Work out the finished part from the listing and answer in its coordinate system (mm). Give positions to 0.01 mm unless a question says otherwise; leave off trailing zeros. Loops run counter-clockwise (first coordinate to the right, second up) from the corner with the lowest first, then second, coordinate; pieces in that order, holes last. Notation, with made-up numbers: M 39,50 L 88,50 A6 cw 88,61 Z; hole C 6.5,1.25 d8. An arc over 180 degrees is marked long. Answer in a Markdown table with one row per item. Add a question column.
from build123d import *

# Parameters (mm, degrees)
F0_R     = 2.5
F0_R_2   = 1.5
F0_R_3   = 11
F1_DEPTH = 5


with BuildPart() as f1:
    # F0 (on Front) → F1 (new body)
    with BuildSketch(Plane.XZ):
        Polygon((-75, -140), (75, -140), (75, 140), (0, 140), (-75, -11.7), align=None)
        with Locations((-40, -120)):
            Circle(F0_R, mode=Mode.SUBTRACT)
        with Locations((-40, -38)):
            Circle(F0_R, mode=Mode.SUBTRACT)
        with Locations((0, -120)):
            Circle(F0_R, mode=Mode.SUBTRACT)
        with Locations((40, -120)):
            Circle(F0_R, mode=Mode.SUBTRACT)
        with Locations((0, -38)):
            Circle(F0_R, mode=Mode.SUBTRACT)
        with Locations((40, -38)):
            Circle(F0_R, mode=Mode.SUBTRACT)
        with Locations((-5.086579, 35.691086)):
            Circle(F0_R_2, mode=Mode.SUBTRACT)
        with Locations((-5.384895, 66.691086)):
            Circle(F0_R_2, mode=Mode.SUBTRACT)
        with Locations((25.913421, 36.207732)):
            Circle(F0_R_2, mode=Mode.SUBTRACT)
        with Locations((30.5, 51.75)):
            Circle(F0_R_3, mode=Mode.SUBTRACT)
        with Locations((25.615105, 67.207732)):
            Circle(F0_R_2, mode=Mode.SUBTRACT)
    extrude(amount=F1_DEPTH)


solid = f1.part
(1) This flat-tipped pin is pushed along its axis until it touches: P1, Ø2, axis at y = -2.5, z = -10.5, coming from the -X side. Where does it stop, or does it pass through?
(2) The mould has two halves that part along Z. Classify faces 1 (the face through (-36.975, -2.465, 65.212)), 2 (the face through (-1, -5, 2)), 3 (the face through (-0.54, -2.46, -40.44)): pulls with the +Z half, pulls with the -Z half, needs draft (parallel to the pull), parting line crosses it, or undercut.
(3) Section C-C, the plane z = 51.75 is taken. Determine the outline of the cut face in (x, y), and give its area (3 significant figures).
(4) Section D-D, the plane x = -15 is taken. Determine the outline of the cut face in (y, z).
(5) Section A-A, the plane x = 30.5 is taken. Determine the outline of the cut face in (y, z), and give its area (3 significant figures).
(6) Section B-B, the plane y = -1.1 is taken. State how many separate pieces and enclosed holes the cut face has, and give its area (3 significant figures).
(7) Consider line 1 along Z through (x, y) = (0, -3.5); line 2 along Z through (x, y) = (42, -4.15); line 3 along Z through (x, y) = (25, -1.15). Determine where each line is inside the solid, lowest interval first. Write a range as from..to.
Numbers:
| question | item | result |
|---|---|---|
| 1 | P1 | stops at x = -74.9 |
| 2 | face 1 | pulls with the +Z half |
| 2 | face 2 | needs draft |
| 2 | face 3 | undercut |
| 3 | outline | M -43.63,-5 L 19.5,-5 L 19.5,0 L -43.63,0 Z; M 41.5,-5 L 75,-5 L 75,0 L 41.5,0 Z |
| 3 | area | 483 mm² |
| 4 | outline | M -5,-140 L 0,-140 L 0,109.66 L -5,109.66 Z |
| 5 | outline | M -5,-140 L 0,-140 L 0,40.75 L -5,40.75 Z; M -5,62.75 L 0,62.75 L 0,140 L -5,140 Z |
| 5 | area | 1,290 mm² |
| 6 | separate pieces | 1 |
| 6 | enclosed holes | 11 |
| 6 | area | 35,800 mm² |
| 7 | line 1 | z = -140..-122.5, -117.5..-40.5, -35.5..140 |
| 7 | line 2 | z = -140..-121.5, -118.5..-39.5, -36.5..140 |
| 7 | line 3 | z = -140..35.02, 37.4..42.22, 61.28..65.84, 68.58..140 |
